CAD build for the part. Positions are in the model's coordinates, mm. Face numbers are marked on the shaded views. A direction names the side the tool comes from. Give positions to 0.01 mm unless a question says otherwise; leave off trailing zeros. Write each loop counter-clockwise with the first axis right and the second up, starting at its lowest first coordinate (ties: lowest second). Pieces come first, ordered by that corner, then holes. Notation, with made-up numbers: M 35,86 L 66,86 A12 cw 66,105 Z; hole C 30,75.25 d1. An arc over 180 degrees is marked long. One line per question, with ' | ' between items. Start each with the question number.
1. Cut at C-C, the plane z = 12.5. Write the cut outline in (x, y), then the cut area to 3 significant figures.
2. Cut at A-A, the plane z = -57.5. Write the cut outline in (x, y), then the cut area to 3 significant figures.
3. Cut at D-D, the plane x = 20. Write the cut outline in (y, z).
4. Cut at B-B, the plane y = 17.5. Write the cut outline in (x, z), then the cut area to 3 significant figures.
5. Wall check: L1, parallel to Z at x = 20, y = -1.75; L2, parallel to Z at x = 32.5, y = 1.5; L3, parallel to Y at x = 3, z = 12. Give the ranges that are in metal, low to high.
6. Pull direction X, two halves, no side cores. Call the marked faces 1, 2 and 3: released by +X, released by -X, zero draft, split by the parting line, or undercut.
7. Which spindle directions (+Z, -Z, +X, -X, +Y, -Y) get a long thin tool onto all of the face, cutting with end or side? Do the marked faces 4, 5 and 6. Say none if no direction does.
8. Flat gauge pins, fed straight in: pin 1 (8 mm diameter, centred on y = -3, z = 14.5, fed in from -X); pin 2 (8 mm diameter, centred on y = -6, z = -53.5, fed in from +X); pin 3 (8 mm diameter, centred on x = 32.5, y = 9.5, fed in from +Z); pin 4 (11 mm diameter, centred on y = 5, z = -57, fed in from -X). Where does each tip first touch, or does it go through?
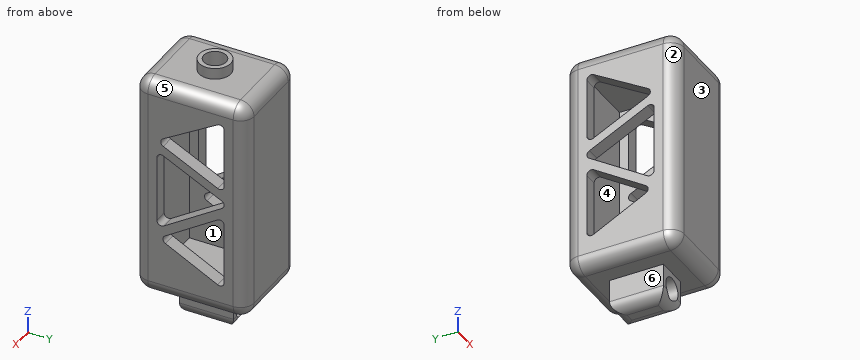
```python
from build123d import *

# Parameters (mm, degrees)
SKETCH1_W           = 100
SKETCH1_H           = 50
BOSS_EXTRUDE1_DEPTH = 40
FILLET1_R           = 6
SKETCH4_R           = 5
CUT_EXTRUDE2_DEPTH  = 8
CUT_EXTRUDE4_DEPTH  = 69.738635424
SKETCH29_W          = 14
SKETCH29_H          = 24
BOSS_EXTRUDE2_DEPTH = 15
SKETCH31_R          = 4.938293982
CUT_EXTRUDE6_DEPTH  = 85.817451035
FILLET7_R           = 5
SKETCH32_W          = 28
SKETCH32_H          = 38
CUT_EXTRUDE7_DEPTH  = 88
BOSS_EXTRUDE3_START = 5
SKETCH33_R          = 7.029692419
SKETCH33_R_2        = 5
BOSS_EXTRUDE3_DEPTH = 5


with BuildPart() as part:
    # Sketch1 → Boss-Extrude1 (new body)
    with BuildSketch(Plane(origin=(0, 0, 0), x_dir=(0, 0, -1), z_dir=(1, 0, 0))):
        Rectangle(SKETCH1_W, SKETCH1_H)
    extrude(amount=BOSS_EXTRUDE1_DEPTH)

    # Fillet1
    fillet1_edges = [part.edges().sort_by_distance(p)[0] for p in [
        (40, 0, 50),
        (40, -25, 0),
        (40, 0, -50),
        (0, -25, 0),
        (0, 0, 50),
        (0, 25, 0),
        (0, 0, -50),
        (20, -25, -50),
        (20, -25, 50),
        (20, 25, 50),
        (20, 25, -50),
        (40, 25, 0),
    ]]
    fillet(fillet1_edges, radius=FILLET1_R)

    # Sketch4 → Cut-Extrude2 (cut)
    with BuildSketch(Plane.XY.offset(50)):
        with Locations((20, 0)):
            Circle(SKETCH4_R)
    extrude(amount=-CUT_EXTRUDE2_DEPTH, mode=Mode.SUBTRACT)

    # Sketch27 → Cut-Extrude4 (cut, through all)
    with BuildSketch(Plane.ZY):
        with BuildLine():
            Line((-35.948740213, 12.085727651), (-23.973812043, -11.212498079))
            ThreePointArc((-23.973812043, -11.212498079), (-22.294505165, -12.295749804), (-20.515873253, -11.384720489))
            Line((-20.515873253, -11.384720489), (-5.440704193, 11.91350524))
            ThreePointArc((-5.440704193, 11.91350524), (-5.363007282, 13.955774681), (-7.119849552, 15))
            Line((-7.119849552, 15), (-34.169946782, 15))
            ThreePointArc((-34.169946782, 15), (-35.877070781, 14.041982558), (-35.948740213, 12.085727651))
        make_face()
        with BuildLine():
            Line((4.169016264, 13.839458065), (17.035163046, -12.111620565))
            ThreePointArc((17.035163046, -12.111620565), (16.94282084, -14.054334181), (15.243297544, -15))
            Line((15.243297544, -15), (-14.291999001, -15))
            ThreePointArc((-14.291999001, -15), (-16.047244937, -13.958703137), (-15.974758786, -11.919111705))
            Line((-15.974758786, -11.919111705), (0.699377924, 14.039691649))
            ThreePointArc((0.699377924, 14.039691649), (2.492379474, 14.947756457), (4.169016264, 13.839458065))
        make_face()
        with BuildLine():
            Line((9.490272401, 12.111620565), (21.518065714, -12.148495172))
            ThreePointArc((21.518065714, -12.148495172), (23.233716027, -13.258663021), (25.028933638, -12.282383156))
            Line((25.028933638, -12.282383156), (39.456095343, 11.977732581))
            ThreePointArc((39.456095343, 11.977732581), (39.475559896, 13.988803611), (37.737092922, 15))
            Line((37.737092922, 15), (11.282137904, 15))
            ThreePointArc((11.282137904, 15), (9.582614607, 14.054334181), (9.490272401, 12.111620565))
        make_face()
    extrude(amount=-CUT_EXTRUDE4_DEPTH, mode=Mode.SUBTRACT)

    # Sketch29 → Boss-Extrude2 (add)
    with BuildSketch(Plane(origin=(0, 0, -50), x_dir=(-1, 0, 0), z_dir=(0, 0, -1))):
        with Locations((-20, 0)):
            Rectangle(SKETCH29_W, SKETCH29_H)
    extrude(amount=BOSS_EXTRUDE2_DEPTH)

    # Sketch31 → Cut-Extrude6 (cut, through all)
    with BuildSketch(Plane.XZ.offset(12)):
        with Locations(Location((20, -57.5, 0), (0, 0, 270))):
            Circle(SKETCH31_R)
    extrude(amount=-CUT_EXTRUDE6_DEPTH, mode=Mode.SUBTRACT)

    # Fillet7
    # the kernel refuses this fillet: 5 mm, written as the material it takes off along each edge
    with BuildSketch(Plane(origin=(13, 24.5, -65), x_dir=(0, 0, 1), z_dir=(0, -1, 0)), Plane(origin=(27, -24.5, -65), x_dir=(0, 0, 1), z_dir=(0, 1, 0))) as fillet7_piece_1:
        with BuildLine():
            CenterArc((FILLET7_R, -FILLET7_R), FILLET7_R, 90, 90)
            Line((0, -FILLET7_R), (0, 0))
            Line((0, 0), (FILLET7_R, 0))
        make_face()
    extrude(amount=49, mode=Mode.SUBTRACT)
    with BuildSketch(Plane(origin=(39.5, 12, -65), x_dir=(0, 0, 1), z_dir=(-1, 0, 0)), Plane(origin=(0.5, -12, -65), x_dir=(0, 0, 1), z_dir=(1, 0, 0))) as fillet7_piece_2:
        with BuildLine():
            CenterArc((FILLET7_R, -FILLET7_R), FILLET7_R, 90, 90)
            Line((0, -FILLET7_R), (0, 0))
            Line((0, 0), (FILLET7_R, 0))
        make_face()
    extrude(amount=39, mode=Mode.SUBTRACT)

    # Sketch32 → Cut-Extrude7 (cut)
    with BuildSketch(Plane.XY.offset(44)):
        with Locations((20, 0)):
            Rectangle(SKETCH32_W, SKETCH32_H)
    extrude(amount=-CUT_EXTRUDE7_DEPTH, mode=Mode.SUBTRACT)

    # Sketch33 → Boss-Extrude3 (add)
    with BuildSketch(Plane.XY.offset(50).offset(BOSS_EXTRUDE3_START)):
        with Locations(Location((20, 0, 0), (0, 0, 90))):
            Circle(SKETCH33_R)
        with Locations((20, 0)):
            Circle(SKETCH33_R_2, mode=Mode.SUBTRACT)
    extrude(amount=-BOSS_EXTRUDE3_DEPTH)


solid = part.part
```
Here are the results:
1) outline: M 0,-19 A6 ccw 6,-25 L 34,-25 A6 ccw 40,-19 L 40,-15 L 34,-15 L 34,-19 L 6,-19 L 6,-15 L 0,-15 Z; M 0,-2.96 L 6,-2.96 L 6,6.04 L 0,6.04 Z; M 0,15 L 6,15 L 6,19 L 34,19 L 34,15 L 40,15 L 40,19 A6 ccw 34,25 L 6,25 A6 ccw 0,19 Z; M 34,-2.96 L 40,-2.96 L 40,6.04 L 34,6.04 Z | area: 653 mm^2
2) outline: M 13,-12 L 15.06,-12 L 15.06,12 L 13,12 Z; M 24.94,-12 L 27,-12 L 27,12 L 24.94,12 Z | area: 99.0 mm^2
3) outline: M -25,-44 A6 ccw -19,-50 L -12,-50 L -12,-52.56 L 12,-52.56 L 12,-50 L 19,-50 A6 ccw 25,-44 L 25,44 A6 ccw 19,50 L 7.03,50 L 7.03,55 L 5,55 L 5,44 L 19,44 L 19,-44 L -19,-44 L -19,44 L -5,44 L -5,55 L -7.03,55 L -7.03,50 L -19,50 A6 ccw -25,44 Z; M -11.37,-62.44 A5 ccw -7,-65 L 7,-65 A5 ccw 11.37,-62.44 Z
4) outline: M 0,-44 A6 ccw 6,-50 L 34,-50 A6 ccw 40,-44 L 40,44 A6 ccw 34,50 L 6,50 A6 ccw 0,44 Z; hole M 6,-44 L 34,-44 L 34,44 L 6,44 Z | area: 1,510 mm^2
5) L1: -65 to -62.44, -52.56 to -44 | L2: -50 to -44, 44 to 50 | L3: -24.2 to -15, -1.96 to 7.05, 15 to 24.2
6) face 1: undercut | face 2: released by -X | face 3: zero draft
7) face 4: none | face 5: +Z, +X, +Y, -Y | face 6: -Z, -X, +Y, -Y
8) pin 1: x = 0 | pin 2: x = 36.4 | pin 3: z = 50 | pin 4: x = 13
